```python
from build123d import *

# Parameters (mm, degrees)
SKETCH1_W            = 180
SKETCH1_H            = 130
BOSS_EXTRUDE1_DEPTH  = 45
SKETCH3_W            = 170
SKETCH3_H            = 120
CUT_EXTRUDE1_DEPTH   = 40
M4_CLEARANCE_HOLE1_D = 4.5
CUT_EXTRUDE2_REACH   = 182
SKETCH7_W            = 18
SKETCH7_H            = 110
SKETCH8_W            = 103
SKETCH8_H            = 18
CUT_EXTRUDE3_DEPTH   = 130


with BuildPart() as part:
    # Sketch1 → Boss-Extrude1 (new body)
    with BuildSketch(Plane.XY):
        Rectangle(SKETCH1_W, SKETCH1_H)
    extrude(amount=BOSS_EXTRUDE1_DEPTH)

    # Sketch3 → Cut-Extrude1 (cut)
    with BuildSketch(Plane.XY):
        Rectangle(SKETCH3_W, SKETCH3_H)
    extrude(amount=CUT_EXTRUDE1_DEPTH, mode=Mode.SUBTRACT)

    # M4 Clearance Hole1 (through all)
    with Locations(Plane(origin=(0, 0, 40), x_dir=(-1, 0, 0), z_dir=(0, 0, -1))):
        with Locations((-23, -48), (70, -48), (70, 48), (-23, 48)):
            Hole(M4_CLEARANCE_HOLE1_D / 2)

    # Sketch7 → Cut-Extrude2 (cut, up to next)
    with BuildSketch(Plane(origin=(90, 0, 0), x_dir=(0, 0, -1), z_dir=(1, 0, 0)), mode=Mode.PRIVATE) as cut_extrude2_sk1:
        with Locations((-9, 0)):
            Rectangle(SKETCH7_W, SKETCH7_H)
    cut_extrude2_tool1 = extrude(cut_extrude2_sk1.sketch, amount=-CUT_EXTRUDE2_REACH, mode=Mode.PRIVATE) & part.part
    add(cut_extrude2_tool1.solids().sort_by_distance((90, 0, 9))[0], mode=Mode.SUBTRACT)

    # Sketch8 → Cut-Extrude3 (cut)
    with BuildSketch(Plane.XZ.offset(65)):
        with Locations((-23.5, 9)):
            Rectangle(SKETCH8_W, SKETCH8_H)
    extrude(amount=-CUT_EXTRUDE3_DEPTH, mode=Mode.SUBTRACT)


solid = part.part
```
Verification items for the finished model (mm, model axes). A direction names the side the tool comes from. Coordinates: 2 decimals unless noted, no trailing zeros. Order: outer loops, then holes, each group sorted by start corner. A loop starts at its lowest first (then second) coordinate and runs counter-clockwise, first axis right, second up. Notation, with made-up numbers: (21, 74) - (59, 74) arc R24 cw to (59, 102) - close; hole circle Ø10 at (-40, -22.75). An arc over 180 degrees is marked (long way). Return JSON: item names as keys, results as strings.
(1) Thickness scan on line 1 along Y through (x, z) = (-70, 43.9); line 2 along Y through (x, z) = (-42, 25); line 3 along X through (y, z) = (-32, 27.5). Record the ranges inside material, lowest first.
Filled sheet:
{"line 1": "y = -65 to -50.25, -45.75 to 45.75, 50.25 to 65", "line 2": "y = -65 to -60, 60 to 65", "line 3": "x = -90 to -85, 85 to 90"}
(2) Section check C-C, the plane z = 8.5. Record the cut outline in (x, y).
Filled sheet:
{"outline": "(-90, -65) - (-75, -65) - (-75, -60) - (-85, -60) - (-85, 60) - (-75, 60) - (-75, 65) - (-90, 65) - close; (28, -65) - (90, -65) - (90, -55) - (85, -55) - (85, -60) - (28, -60) - close; (28, 60) - (85, 60) - (85, 55) - (90, 55) - (90, 65) - (28, 65) - close"}
(3) Section check B-B, the plane x = 23. Record the cut outline in (y, z), and give its area (3 significant figures).
Filled sheet:
{"outline": "(-65, 18) - (-60, 18) - (-60, 40) - (-50.25, 40) - (-50.25, 45) - (-65, 45) - close; (-45.75, 40) - (45.75, 40) - (45.75, 45) - (-45.75, 45) - close; (50.25, 40) - (60, 40) - (60, 18) - (65, 18) - (65, 45) - (50.25, 45) - close", "area": "825 mm^2"}
(4) Mould release check, pull along X, two halves, no side actions. Record for faces 1 (the flat face through (90, -1, 27)), 2 (the flat face through (-1, 1, 40)), 3 (the flat face through (88, -55, 9)): pulls with the +X half, pulls with the -X half, needs draft (parallel to the pull), parting line crosses it, or undercut.
Filled sheet:
{"face 1": "pulls with the +X half", "face 2": "undercut", "face 3": "needs draft"}
(5) Access from +Z, -Z, +X, -X, +Y, -Y to the whole of each face (thin tool, end or side, straight path). Record for faces 4 (the cylindrical face through (-68.79, -46.103, 42.535)), 5 (the flat face through (-85, -1, 20)), 6 (the flat face through (59, 62, 0)), 7 (the flat face through (-75, -63, 9)), 8 (the flat face through (88, 55, 9)).
Filled sheet:
{"face 4": "+Z, -Z", "face 5": "-Z", "face 6": "-Z, +X, -X, +Y, -Y", "face 7": "-Z, +Y, -Y", "face 8": "-Z, +X"}
(6) Section check A-A, the plane y = 48. Record the cut outline in (x, z).
Filled sheet:
{"outline": "(-90, 0) - (-85, 0) - (-85, 40) - (-72.25, 40) - (-72.25, 45) - (-90, 45) - close; (-67.75, 40) - (20.75, 40) - (20.75, 45) - (-67.75, 45) - close; (25.25, 40) - (85, 40) - (85, 18) - (90, 18) - (90, 45) - (25.25, 45) - close"}
(7) Go/stop test with flat-tipped pins: pin 1 (1 mm diameter, centred on x = -60, y = -7, fed in from -Z); pin 2 (1.5 mm diameter, centred on y = -13, z = 16, fed in from +X); pin 3 (5.5 mm diameter, centred on x = -35.5, y = -61.5, fed in from -Z). Record where each tip stops, or that it passes through.
Filled sheet:
{"pin 1": "stops at z = 40", "pin 2": "stops at x = -85", "pin 3": "stops at z = 18"}
(8) Section check D-D, the plane z = 28. Record the cut outline in (x, y), and give its area (3 significant figures).
Filled sheet:
{"outline": "(-90, -65) - (90, -65) - (90, 65) - (-90, 65) - close; hole (-85, -60) - (85, -60) - (85, 60) - (-85, 60) - close", "area": "3,000 mm^2"}
